```python
from build123d import *

# Parameters (mm, degrees)
SKETCH1_W           = 12.7
SKETCH1_H           = 18.986000128
SKETCH1_R           = 1.75
BOSS_EXTRUDE1_DEPTH = 3.048
SKETCH3_W           = 21.59
SKETCH3_H           = 3.81
BOSS_EXTRUDE2_DEPTH = 12.7
SKETCH4_R           = 2
CUT_EXTRUDE1_DEPTH  = 32.746208354


with BuildPart() as part:
    # Sketch1 → Boss-Extrude1 (new body)
    with BuildSketch(Plane.XY):
        Rectangle(SKETCH1_W, SKETCH1_H)
        with Locations(Location((0, -5.203000064, 0), (0, 0, 180))):
            Circle(SKETCH1_R, mode=Mode.SUBTRACT)
    extrude(amount=BOSS_EXTRUDE1_DEPTH)

    # Sketch3 → Boss-Extrude2 (add, through all)
    with BuildSketch(Plane(origin=(6.35, 0, 0), x_dir=(0, 0, -1), z_dir=(1, 0, 0))):
        with Locations((-13.843, 7.588000064)):
            Rectangle(SKETCH3_W, SKETCH3_H)
    extrude(amount=-BOSS_EXTRUDE2_DEPTH)

    # Sketch4 → Cut-Extrude1 (cut, through all)
    with BuildSketch(Plane(origin=(0, 9.493000064, 0), x_dir=(1, 0, 0), z_dir=(0, 1, 0))):
        with Locations(Location((0, -20.828, 0), (0, 0, 270))):
            Circle(SKETCH4_R)
        with Locations((0, -5.588)):
            Circle(SKETCH4_R)
    extrude(amount=-CUT_EXTRUDE1_DEPTH, mode=Mode.SUBTRACT)


solid = part.part
```
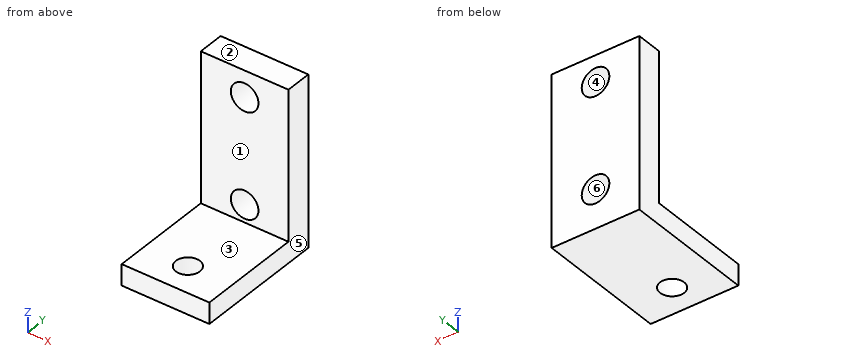
Geometry: final body of the model. Coordinates: model frame, mm. Face numbers are marked on the shaded views. A direction names the side the tool comes from. Round coordinates to 2 decimals unless told otherwise and drop trailing zeros. Loops run counter-clockwise (first coordinate to the right, second up) from the corner with the lowest first, then second, coordinate; pieces in that order, holes last. Notation, with made-up numbers: (2.5, -29.5) -> (15.5, -29.5) arc R16 ccw to (15.5, -1.5) -> close; hole circle Ø11 at (-25, 77). An arc over 180 degrees is marked (long way). Write each question's results on one line, items separated by ' | '.
Item 1: Cut plane D-D on x = -5.5. Return the cut outline in (y, z), and give its area (3 significant figures).
Answers below:
outline: (-9.49, 0) -> (9.49, 0) -> (9.49, 24.64) -> (5.68, 24.64) -> (5.68, 3.05) -> (-9.49, 3.05) -> close | area: 140 mm²
Item 2: Cut plane C-C on z = 7. Return the cut outline in (x, y).
Answers below:
outline: (-6.35, 5.68) -> (-1.42, 5.68) -> (-1.42, 9.49) -> (-6.35, 9.49) -> close; (1.42, 5.68) -> (6.35, 5.68) -> (6.35, 9.49) -> (1.42, 9.49) -> close
Item 3: Line query: probe 1 along Y at (x, z) = (0, 1.35); probe 2 along Z at (x, y) = (1.25, 8); probe 3 along Y at (x, z) = (-3.5, 10). Output: solid intervals per line, ascending. Write a range as [from, to].
Answers below:
probe 1: y = [-9.49, -6.95], [-3.45, 9.49] | probe 2: z = [0, 4.03], [7.15, 19.27], [22.39, 24.64] | probe 3: y = [5.68, 9.49]
Item 4: Cut plane B-B on y = -6. Return the cut outline in (x, z).
Answers below:
outline: (-6.35, 0) -> (-1.56, 0) -> (-1.56, 3.05) -> (-6.35, 3.05) -> close; (1.56, 0) -> (6.35, 0) -> (6.35, 3.05) -> (1.56, 3.05) -> close
Item 5: Pull-direction query (Z, two-part tool) for the marked faces 3, 4, 5 and 6; classes: pulls with the +Z half, pulls with the -Z half, needs draft (parallel to the pull), parting line crosses it, or undercut.
Answers below:
face 3: pulls with the +Z half | face 4: undercut | face 5: needs draft | face 6: undercut
Item 6: Set-up query: the marked faces 1 and 2. Return all of +Z, -Z, +X, -X, +Y, -Y with unobstructed straight access to the full face (end or side cutting, diameter ignored); none if empty.
Answers below:
face 1: +Z, +X, -X, -Y | face 2: +Z, +X, -X, +Y, -Y
Item 7: Cut plane A-A on x = 0. Return the cut outline in (y, z).
Answers below:
outline: (-9.49, 0) -> (-6.95, 0) -> (-6.95, 3.05) -> (-9.49, 3.05) -> close; (-3.45, 0) -> (9.49, 0) -> (9.49, 3.59) -> (5.68, 3.59) -> (5.68, 3.05) -> (-3.45, 3.05) -> close; (5.68, 7.59) -> (9.49, 7.59) -> (9.49, 18.83) -> (5.68, 18.83) -> close; (5.68, 22.83) -> (9.49, 22.83) -> (9.49, 24.64) -> (5.68, 24.64) -> close
Item 8: Pin query (flat end, axial travel): pin 1 Ø3 at (x, y) = (3, 1) entering from +Z; pin 2 Ø4.5 at (x, z) = (0, 20.828) entering from -Y; pin 3 Ø3 at (x, z) = (0, 5.588) entering from +Y. Return the tip coordinate at first contact, or that it passes through.
Answers below:
pin 1: stops at z = 3.05 | pin 2: stops at y = 5.68 | pin 3: passes through
